Design review of the part shown in the three views and the two pictorial views. Dimensions are in mm from the part's minimum x, y and z. A direction names the side the tool comes from. Give positions to 0.01 mm unless a question says otherwise; leave off trailing zeros. Loops run counter-clockwise (first coordinate to the right, second up) from the corner with the lowest first, then second, coordinate; pieces in that order, holes last. Notation, with made-up numbers: (10.25, 30.5) - (50.25, 30.5) arc R28 ccw to (50.25, 58.5) - close; hole circle Ø11 at (-34.75, -14.75). An arc over 180 degrees is marked (long way). Answer in a Markdown table with one row per item.
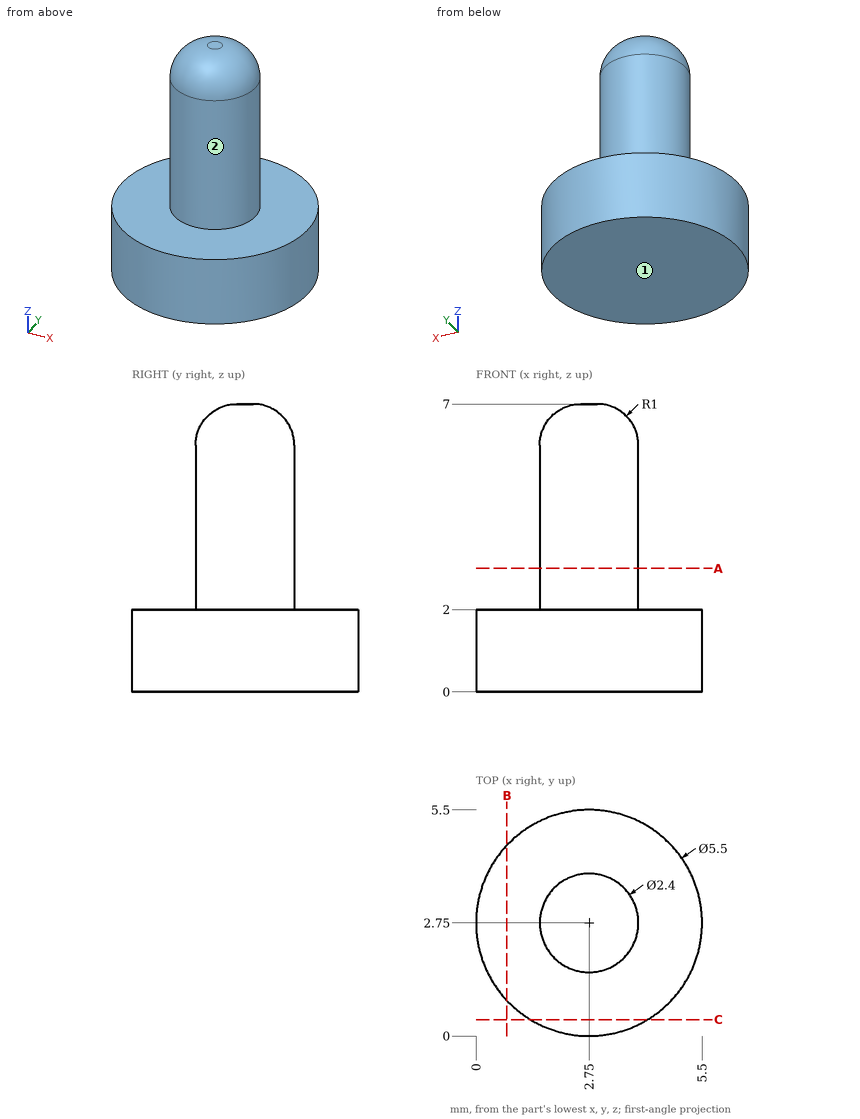
1. We need section A-A, the plane z = 3. Give the boundary of the cut face in (x, y), and give its area (3 significant figures).
Values:
| item | result |
|---|---|
| outline | circle Ø2.4 at (2.75, 2.75) |
| area | 4.52 mm^2 |
2. We need section B-B, the plane x = 0.75. Give the boundary of the cut face in (y, z).
Values:
| item | result |
|---|---|
| outline | (0.86, 0) - (4.64, 0) - (4.64, 2) - (0.86, 2) - close |
3. Clearance check with flat-ended pins moving along their axes: pin 1 (1.5 mm diameter, centred on y = 1.5, z = 3, fed in from +X); pin 2 (3 mm diameter, centred on x = 4.5, z = 2, fed in from -Y). State where each tip first meets the part, or that it passes through.
Values:
| item | result |
|---|---|
| pin 1 | stops at x = 3.84 |
| pin 2 | stops at y = 0.01 |
4. For the marked faces 1 and 2, list the 3-axis set-ups (+Z, -Z, +X, -X, +Y, -Y) from which the entire face can be reached by the end or side of a thin tool; tool diameter is ignored.
Values:
| item | result |
|---|---|
| face 1 | -Z, +X, -X, +Y, -Y |
| face 2 | +Z |
5. We need section C-C, the plane y = 0.4. Give the boundary of the cut face in (x, z).
Values:
| item | result |
|---|---|
| outline | (1.32, 0) - (4.18, 0) - (4.18, 2) - (1.32, 2) - close |
6. Wall thickness on line 1 (Z direction, x = 2.8, y = 1.1); line 2 (Z direction, x = 3.6, y = 3.25); line 3 (Y direction, x = 5.2, z = 0.5): over which ranges is each line inside the solid? List them lowest first. Write a range as [from, to].
Values:
| item | result |
|---|---|
| line 1 | z = [0, 2] |
| line 2 | z = [0, 6.62] |
| line 3 | y = [1.5, 4] |
